Study the drawing (mm; zero at the part's minimum x, y, z) and answer. A direction names the side the tool comes from. Coordinates: 2 decimals unless noted, no trailing zeros. Loops run counter-clockwise (first coordinate to the right, second up) from the corner with the lowest first, then second, coordinate; pieces in that order, holes last. Notation, with made-up numbers: (61, 38.5) - (103, 38.5) arc R19 ccw to (103, 63.5) - close; hole circle Ø9 at (4, 71.25). An arc over 180 degrees is marked (long way). Use one line per item in the form item = value. Start each with the question number.
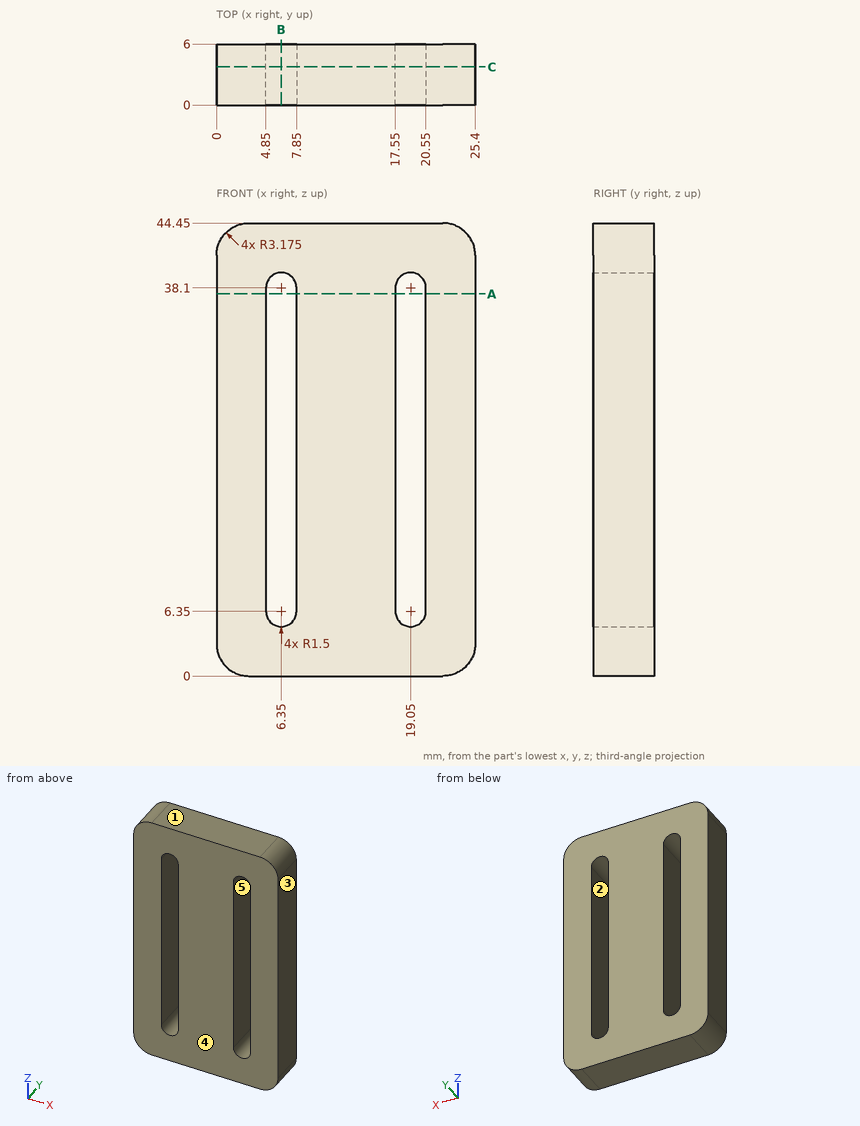
(1) Find the intervals of material crossed by probe 1 along X at (y, z) = (1.05, 25); probe 2 along Z at (x, y) = (6.25, 1.55); probe 3 along X at (y, z) = (3.9, 5.5), in increasing order. Write a range as from..to.
(2) For the marked faces 4 and 5, determine the directions among +Z, -Z, +X, -X, +Y, -Y from which every point of the face is accessible in a straight line to the end or side of a thin tool.
(3) A cutting plane is placed at B-B (x = 6.35). Determine the outline of the cut face in (y, z).
(4) This flat-tipped pin is pushed along its axis until it touches: pin 1 Ø2 at (x, y) = (6.5, 1.5) entering from -Z. Where does it stop, or does it pass through?
(5) Determine the mould class of the marked faces 1, 2 and 3 for opening direction X: +X half, -X half, draft (parallel to the pull), parting line (faces both ways), or undercut.
(6) A cutting plane is placed at A-A (z = 37.5). Determine the outline of the cut face in (x, y), then the cut area to 3 significant figures.
(7) A cutting plane is placed at C-C (y = 3.75). Determine the outline of the cut face in (x, z) (3 decimals), then the cut area to 3 significant figures.
Evaluation:
q1.probe_1 = 0..4.85, 7.85..17.55, 20.55..25.4
q1.probe_2 = 0..4.85, 39.6..44.45
q1.probe_3 = 0..5.11, 7.59..17.81, 20.29..25.4
q2.face_4 = +Z, -Z, +X, -X, -Y
q2.face_5 = +Y, -Y
q3.outline = (0, 0) - (6, 0) - (6, 4.85) - (0, 4.85) - close; (0, 39.6) - (6, 39.6) - (6, 44.45) - (0, 44.45) - close
q4.pin_1 = 0
q5.face_1 = draft
q5.face_2 = undercut
q5.face_3 = +X half
q6.outline = (0, 0) - (4.85, 0) - (4.85, 6) - (0, 6) - close; (7.85, 0) - (17.55, 0) - (17.55, 6) - (7.85, 6) - close; (20.55, 0) - (25.4, 0) - (25.4, 6) - (20.55, 6) - close
q6.area = 116 mm^2
q7.outline = (0, 3.175) arc R3.175 ccw to (3.175, 0) - (22.225, 0) arc R3.175 ccw to (25.4, 3.175) - (25.4, 41.275) arc R3.175 ccw to (22.225, 44.45) - (3.175, 44.45) arc R3.175 ccw to (0, 41.275) - close; hole (4.85, 6.35) arc R1.5 ccw to (7.85, 6.35) - (7.85, 38.1) arc R1.5 ccw to (4.85, 38.1) - close; hole (17.55, 6.35) arc R1.5 ccw to (20.55, 6.35) - (20.55, 38.1) arc R1.5 ccw to (17.55, 38.1) - close
q7.area = 916 mm^2
